Geometry check sheet. Reference: drawing and pictorial views, mm from the part's lowest x, y, z. A direction names the side the tool comes from. Round coordinates to 2 decimals unless told otherwise and drop trailing zeros. Loops run counter-clockwise (first coordinate to the right, second up) from the corner with the lowest first, then second, coordinate; pieces in that order, holes last. Notation, with made-up numbers: (84.25, 56.5) - (110.25, 56.5) arc R30 cw to (110.25, 90.5) - close; hole circle Ø1 at (0, 64.25). An arc over 180 degrees is marked (long way). Answer as CSV lines item,"result". Start each with the question number.
1) Depth check by flat-ended pin: P1, Ø5, axis at y = 2, z = 44.5, coming from the -X side; P2, Ø2, axis at x = 20, y = 8, coming from the -Z side; P3, Ø4, axis at y = 10, z = 40, coming from the +X side. Enter the tip coordinate at first touch or a pass-through.
2) Cross-section at B-B on y = 7.25. Record the boundary of the cut face in (x, z) (1 decimal), and give its area (3 significant figures).
3) Cross-section at C-C on z = 35. Record the boundary of the cut face in (x, y).
4) Cross-section at D-D on x = 30. Record the boundary of the cut face in (y, z) (1 decimal).
5) Cross-section at A-A on x = 11.5. Record the boundary of the cut face in (y, z), and give its area (3 significant figures).
6) Thickness scan on line 1 along Z through (x, y) = (26, 4.5) (1 decimal); line 2 along Z through (x, y) = (23, 3.25) (1 decimal); line 3 along X through (y, z) = (6, 42). Record the ranges inside material, lowest first.
7) Access from +Z, -Z, +X, -X, +Y, -Y to the whole of each face (thin tool, end or side, straight path). Record for the marked faces 1, 2 and 3.
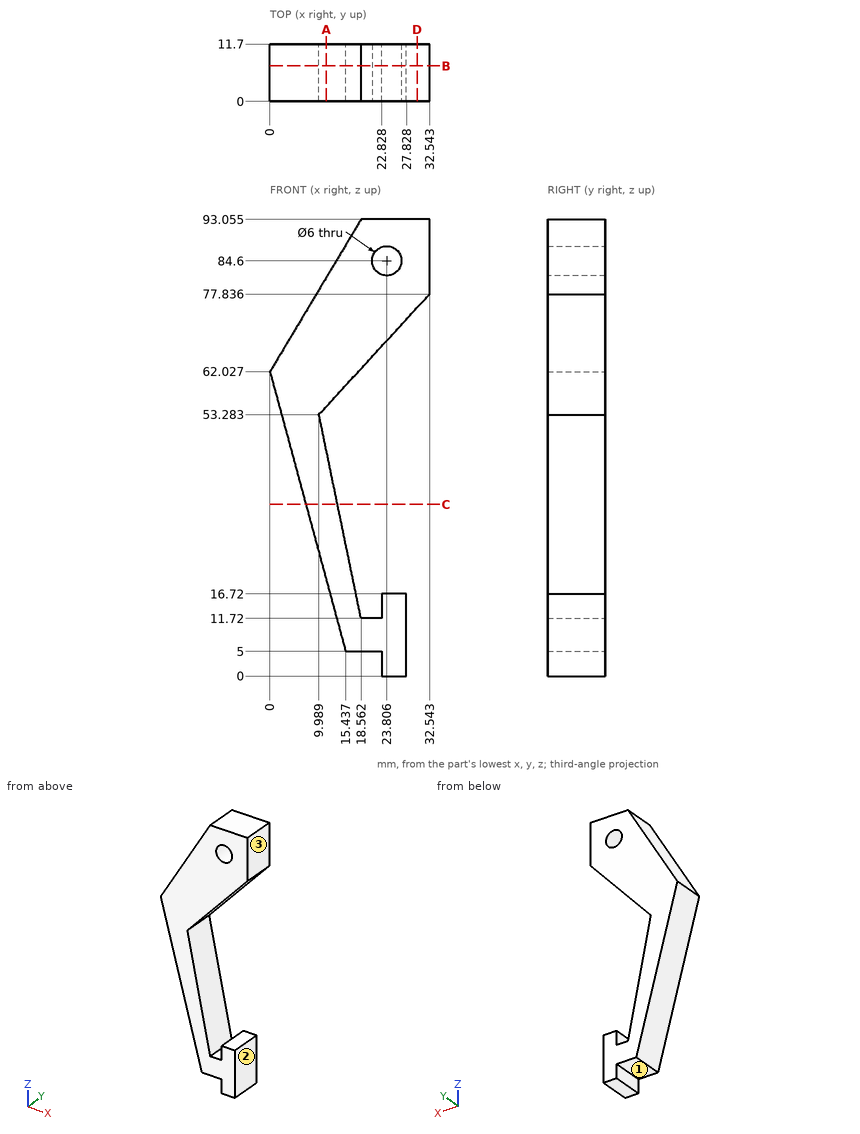
Answer block:
1,P1,"stops at x = 4.07"
1,P2,"stops at z = 5"
1,P3,"stops at x = 13.14"
2,outline,"(0, 62) - (15.4, 5) - (22.8, 5) - (22.8, 0) - (27.8, 0) - (27.8, 16.7) - (22.8, 16.7) - (22.8, 11.7) - (18.6, 11.7) - (10, 53.3) - (32.5, 77.8) - (32.5, 93.1) - (18.6, 93.1) - close; hole circle Ø6 at (23.8, 84.6)"
2,area,"1,090 mm^2"
3,outline,"(7.32, 0) - (13.76, 0) - (13.76, 11.7) - (7.32, 11.7) - close"
4,outline,"(0, 75.1) - (11.7, 75.1) - (11.7, 93.1) - (0, 93.1) - close"
5,outline,"(0, 19.54) - (11.7, 19.54) - (11.7, 45.96) - (0, 45.96) - close; (0, 54.93) - (11.7, 54.93) - (11.7, 81.25) - (0, 81.25) - close"
5,area,"617 mm^2"
6,line 1,"z = 0 to 16.7, 70.7 to 82.6, 86.6 to 93.1"
6,line 2,"z = 0 to 16.7, 67.4 to 81.7, 87.5 to 93.1"
6,line 3,"x = 5.42 to 12.32"
7,face 1,"-Z, -X, +Y, -Y"
7,face 2,"-Z, +X, +Y, -Y"
7,face 3,"+Z, -Z, +X, +Y, -Y"
